Autodesk Inventor part; units mm, degrees
ref_plane "bolt_to_nut_XY" through (35, 0, 0) normal (1, 0, 0) x (0, 0, -1)
ref_plane "bolt_to_nut_YZ" through (35, 0, 0) normal (0, 0, -1) x (0, 1, 0)
ref_plane "bolt_to_nut_ZX" through (35, 0, 0) normal (0, 1, 0) x (1, 0, 0)
sketch "Sketch_2" plane through (0, 0, 0) normal (0, 0, 1) x (1, 0, 0)
  line L0 (35, 0) -> (-5, 0)
  line L1 (-5, 0) -> (-5, 3.75)
  line L2 (-5, 3.75) -> (-4.5, 4.25)
  line L3 (-4.5, 4.25) -> (0, 4.25)
  line L4 (0, 4.25) -> (0, 2.5)
  line L5 (0, 2.5) -> (34.5095, 2.5)
  line L6 (34.5095, 2.5) -> (35, 2.0095)
  line L7 (35, 2.0095) -> (35, 0)
  line L8 (35, 0) -> (-5, 0)
revolve "Revolution1" add sketch "Sketch_2" angle 360 about axis through (35, 0, 0) along (1, 0, 0)
thread "Thread1"
sketch "Sketch2" plane through (-5, 0, 0) normal (-1, 0, 0) x (0, 0, 1)
  point P0 (0, 0)
hole "Hole1" at (-5, 0, 0) direction (1, 0, 0) diameter 4 depth 2.5 tip angle 150
sketch "Sketch_3" plane through (-5, 0, 0) normal (1, 0, 0) x (0, 0, -1)
  line L0 (-2, -1.1547) -> (0, -2.3094)
  line L1 (0, -2.3094) -> (2, -1.1547)
  line L2 (2, -1.1547) -> (2, 1.1547)
  line L3 (2, 1.1547) -> (0, 2.3094)
  line L4 (0, 2.3094) -> (-2, 1.1547)
  line L5 (-2, 1.1547) -> (-2, -1.1547)
extrude "Extrusion1" cut sketch "Sketch_3" along normal blind 2.5
ref_plane "bolt_to_nut_XY" through (35, 0, 0) normal (1, 0, 0) x (0, 0, -1)
ref_plane "bolt_to_nut_YZ" through (35, 0, 0) normal (0, 0, -1) x (0, 1, 0)
ref_plane "bolt_to_nut_ZX" through (35, 0, 0) normal (0, 1, 0) x (1, 0, 0)
ref_plane "screw1_XY" through (0, 0, 0) normal (1, 0, 0) x (0, 0, -1)
ref_plane "screw1_YZ" through (0, 0, 0) normal (0, 0, -1) x (0, 1, 0)
ref_plane "screw1_ZX" through (0, 0, 0) normal (0, 1, 0) x (1, 0, 0)
properties part number "CB5-35"
For this review, take the finished solid that the model builds, in its own axes (mm). A direction names the side the tool comes from. Round coordinates to 2 decimals unless told otherwise and drop trailing zeros. Write each loop counter-clockwise with the first axis right and the second up, starting at its lowest first coordinate (ties: lowest second). Pieces come first, ordered by that corner, then holes. Notation, with made-up numbers: (18, 73.25) -> (31, 73.25) arc R26 cw to (31, 108.25) -> close; hole circle Ø11 at (80, 7.5). An arc over 180 degrees is marked (long way). Use one line per item in the form item = value.
1) Mouldability with a two-part tool opening along Z and no side actions: class faces 1 (the cylindrical face through (17.5, -0.54, -2.44)), 2 (the flat face through (0, 2, -2)), 3 (the flat face through (-4, 0, 2)) as +Z half, -Z half, draft (parallel to the pull), parting line (faces both ways), or undercut.
Found:
face_1 = parting line
face_2 = draft
face_3 = undercut
2) Tool access review of faces 4 (the cylindrical face through (-2.218, 2.285, 3.584)), 5 (the flat face through (-3.77, -1.74, -0.99)): name each direction out of +Z, -Z, +X, -X, +Y, -Y from which nothing blocks a thin tool from reaching the whole face with its end or side.
Found:
face_4 = +X, -X
face_5 = -X
3) Take a section at A-A, the plane x = 31. Write out the cut boundary in (y, z).
Found:
outline = circle Ø5 at (0, 0)
4) To check wall thickness, follow L1, parallel to Y at x = 7, z = -1.5; L2, parallel to X at y = 2.5, z = 1.5; L3, parallel to Z at x = 13.5, y = 0. State the ranges of each line that lie inside material, in increasing order. Write a range as from..to.
Found:
L1 = -2..2
L2 = -5..0
L3 = -2.5..2.5
5) Clearance check with flat-ended pins moving along their axes: pin 1 (1 mm diameter, centred on x = 10, y = 2, fed in from +Z); pin 2 (1.5 mm diameter, centred on x = 24, y = -1, fed in from +Z); pin 3 (1.5 mm diameter, centred on x = 7.5, z = -2.5, fed in from -Y); pin 4 (2.5 mm diameter, centred on x = -3.5, y = -0.5, fed in from -Z). State where each tip first meets the part, or that it passes through.
Found:
pin_1 = 2
pin_2 = 2.49
pin_3 = -1.79
pin_4 = -4.25
